Design review of the part built by this model. Coordinates are the model's own, in mm. Coordinates: 2 decimals unless noted, no trailing zeros. Order: outer loops, then holes, each group sorted by start corner. A loop starts at its lowest first (then second) coordinate and runs counter-clockwise, first axis right, second up.
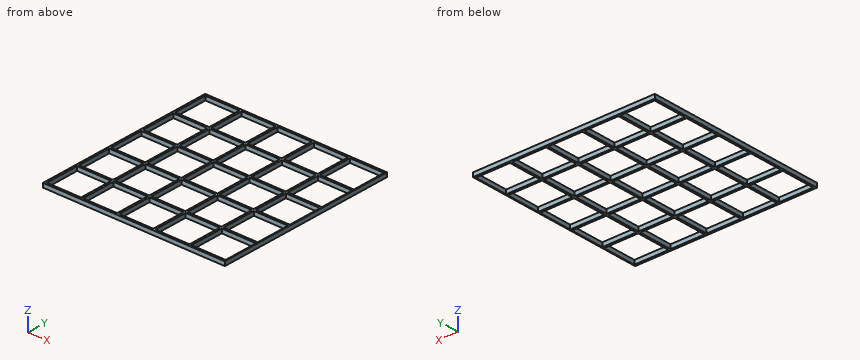
from build123d import *

# Parameters (mm, degrees)
CROQUIS1_W              = 37
CROQUIS1_H              = 37
CROQUIS1_W_2            = 33
CROQUIS1_H_2            = 33
SALIENTE_EXTRUIR1_DEPTH = 4
MATRIZL1_COUNT          = 5
MATRIZL1_PITCH          = 35
MATRIZL1_COUNT_DIR2     = 5
MATRIZL1_PITCH_DIR2     = 35
CROQUIS2_W              = 1
CROQUIS2_H              = 177
CORTAR_EXTRUIR1_DEPTH   = 10


with BuildPart() as part:
    # Croquis1 → Saliente-Extruir1 (new body)
    with BuildSketch(Plane.XY):
        with Locations((17.5, -17.5)):
            Rectangle(CROQUIS1_W, CROQUIS1_H)
        with Locations((17.5, -17.5)):
            Rectangle(CROQUIS1_W_2, CROQUIS1_H_2, mode=Mode.SUBTRACT)
    saliente_extruir1 = extrude(amount=SALIENTE_EXTRUIR1_DEPTH)

    # MatrizL1: Saliente-Extruir1 5 × 5
    with Locations(*[(-i * MATRIZL1_PITCH, j * MATRIZL1_PITCH_DIR2, 0) for i in range(MATRIZL1_COUNT) for j in range(MATRIZL1_COUNT_DIR2) if (i, j) != (0, 0)]):
        add(saliente_extruir1)

    # Croquis2 → Cortar-Extruir1 (cut)
    with BuildSketch(Plane.XY.offset(4)):
        with Locations((35.5, 52.5)):
            Rectangle(CROQUIS2_W, CROQUIS2_H)
    extrude(amount=-CORTAR_EXTRUIR1_DEPTH, mode=Mode.SUBTRACT)


solid = part.part
1. Add section B-B (y = 64). Give the boundary of the cut face in (x, z).
2. To check wall thickness, follow line 1 (Y direction, x = -27.5, z = 3.3); line 2 (X direction, y = -16, z = 2.05). State the ranges of each line that lie inside material, in increasing order.
3. Add section A-A (x = -12.5). Give the boundary of the cut face in (y, z), and give its area (3 significant figures).
4. Add section C-C (z = 1.65). State how many separate pieces and enclosed holes the cut face has, and give its area (3 significant figures).
Solution:
1. outline: (-141, 0) - (-139, 0) - (-139, 4) - (-141, 4) - close; (-106, 0) - (-104, 0) - (-104, 4) - (-106, 4) - close; (-71, 0) - (-69, 0) - (-69, 4) - (-71, 4) - close; (-36, 0) - (-34, 0) - (-34, 4) - (-36, 4) - close; (-1, 0) - (1, 0) - (1, 4) - (-1, 4) - close; (34, 0) - (35, 0) - (35, 4) - (34, 4) - close
2. line 1: y = -36 to -34, -1 to 1, 34 to 36, 69 to 71, 104 to 106, 139 to 141
2. line 2: x = -141 to -139, -106 to -104, -71 to -69, -36 to -34, -1 to 1, 34 to 35
3. outline: (-36, 0) - (-34, 0) - (-34, 4) - (-36, 4) - close; (-1, 0) - (1, 0) - (1, 4) - (-1, 4) - close; (34, 0) - (36, 0) - (36, 4) - (34, 4) - close; (69, 0) - (71, 0) - (71, 4) - (69, 4) - close; (104, 0) - (106, 0) - (106, 4) - (104, 4) - close; (139, 0) - (141, 0) - (141, 4) - (139, 4) - close
3. area: 48.0 mm2
4. separate pieces: 1
4. enclosed holes: 25
4. area: 3,930 mm2
